Design review of the part built by this model. Coordinates are the model's own, in mm. A direction names the side the tool comes from. Coordinates: 2 decimals unless noted, no trailing zeros. Loops run counter-clockwise (first coordinate to the right, second up) from the corner with the lowest first, then second, coordinate; pieces in that order, holes last. Notation, with made-up numbers: (33.25, 21) -> (45.25, 21) arc R25 cw to (45.25, 46) -> close; hole circle Ø3 at (-21, 30.25). An arc over 180 degrees is marked (long way). Use CSV: the item, a comma, the result in double quotes.
```python
from build123d import *

# Parameters (mm, degrees)
SKETCH1_R           = 12.7
SKETCH1_R_2         = 2
BOSS_EXTRUDE1_DEPTH = 12.7
SKETCH2_W           = 38.1
SKETCH2_H           = 76.2
BOSS_EXTRUDE2_DEPTH = 12.7
FILLET1_R           = 12.7
SKETCH3_W           = 6.35
SKETCH3_H           = 31.75
CUT_EXTRUDE1_DEPTH  = 89.9
BOSS_EXTRUDE3_DEPTH = 38.1
FILLET2_R           = 3.175


with BuildPart() as part:
    # Sketch1 → Boss-Extrude1 (new body)
    # profile 1 of 2: a face of its own
    with BuildSketch(Plane.XY):
        Circle(SKETCH1_R)
        Circle(SKETCH1_R_2, mode=Mode.SUBTRACT)
    # profile 2 of 2: a face of its own
    with BuildSketch(Plane.XY):
        with BuildLine():
            ThreePointArc((12.7, 0), (8.980256121, -8.980256121), (0, -12.7))
            Line((0, -12.7), (25.4, -12.7))
            Line((25.4, -12.7), (25.4, 12.7))
            Line((25.4, 12.7), (0, 12.7))
            ThreePointArc((0, 12.7), (8.980256121, 8.980256121), (12.7, 0))
        make_face()
    extrude(amount=BOSS_EXTRUDE1_DEPTH)

    # Sketch2 → Boss-Extrude2 (add)
    with BuildSketch(Plane(origin=(25.4, 0, 0), x_dir=(0, 0, -1), z_dir=(1, 0, 0))):
        with Locations((-6.35, 0)):
            Rectangle(SKETCH2_W, SKETCH2_H)
    extrude(amount=BOSS_EXTRUDE2_DEPTH)

    # Fillet1
    fillet1_edges = [part.edges().sort_by_distance(p)[0] for p in [
        (25.4, 12.7, 6.35),
        (25.4, -12.7, 6.35),
        (25.4, 0, 12.7),
        (25.4, 0, 0),
    ]]
    fillet(fillet1_edges, radius=FILLET1_R - 0.0001)  # a hair under: the kernel refuses the full size

    # Sketch3 → Cut-Extrude1 (cut, through all)
    with BuildSketch(Plane(origin=(0, 38.1, 0), x_dir=(1, 0, 0), z_dir=(0, 1, 0))):
        with Locations((31.75, -6.35)):
            Rectangle(SKETCH3_W, SKETCH3_H)
    extrude(amount=-CUT_EXTRUDE1_DEPTH, mode=Mode.SUBTRACT)

    # Sketch4 → Boss-Extrude3 (add)
    with BuildSketch(Plane.XY.offset(25.4)):
        with BuildLine():
            Line((38.1, 38.1), (38.1, 25.4))
            ThreePointArc((38.1, 25.4), (44.45, 31.75), (38.1, 38.1))
        make_face()
        with BuildLine():
            Line((38.1, -25.4), (38.1, -38.1))
            ThreePointArc((38.1, -38.1), (44.45, -31.75), (38.1, -25.4))
        make_face()
    extrude(amount=-BOSS_EXTRUDE3_DEPTH)

    # Fillet2
    fillet2_edges = [part.edges().sort_by_distance(p)[0] for p in [
        (34.925, 0, 22.225),
        (28.575, 0, 22.225),
        (34.925, 0, -9.525),
        (28.575, 0, -9.525),
        (38.1, 0, 25.4),
        (38.1, 0, -12.7),
    ]]
    fillet(fillet2_edges, radius=FILLET2_R - 0.0001)  # a hair under: the kernel refuses the full size


solid = part.part
```
Item 1: Add section B-B (y = 0). State how many separate pieces and enclosed holes the cut face has, then the cut area to 3 significant figures.
Checked values:
separate pieces,"2"
enclosed holes,"1"
area,"789 mm^2"
Item 2: To check wall thickness, follow line 1 along X through (y, z) = (18, 3.5) (3 decimals); line 2 along X through (y, z) = (-5, 7) (3 decimals); line 3 along Y through (x, z) = (41.5, 0). State the ranges of each line that lie inside material, in increasing order.
Checked values:
line 1,"23.021 to 28.575, 34.925 to 38.1"
line 2,"-11.674 to 28.575, 34.925 to 38.1"
line 3,"-37.11 to -26.39, 26.39 to 37.11"
Item 3: Add section A-A (z = 3). Give the boundary of the cut face in (x, y) (3 decimals).
Checked values:
outline,"(0, -12.7) -> (12.7, -12.7) arc R12.7 cw to (25.4, -25.4) -> (25.4, -38.1) -> (28.575, -38.1) -> (28.575, 38.1) -> (25.4, 38.1) -> (25.4, 25.4) arc R12.7 cw to (12.7, 12.7) -> (0, 12.7) arc R12.7 ccw to start; (34.925, -38.1) -> (38.1, -38.1) arc R6.35 ccw to (38.1, -25.4) -> (38.1, 25.4) arc R6.35 ccw to (38.1, 38.1) -> (34.925, 38.1) -> close; hole circle Ø4 at (0, 0)"
Item 4: Machinability: for faces 1 (the face through (38.1, 0, 7)), 2 (the face through (33.97, -0.53, 21.32)), 3 (the face through (6, 12.7, 6)), 4 (the face through (6, -12.7, 6)), which of the approach directions +Z, -Z, +X, -X, +Y, -Y give a long, thin tool a straight path to every point of the face, cutting with its end or side? Answer none if there is none.
Checked values:
face 1,"+Z, -Z, +X"
face 2,"+Y, -Y"
face 3,"+Z, -Z, -X, +Y"
face 4,"+Z, -Z, -X, -Y"
Item 5: Draft analysis for pull direction Z (two halves, no side actions). For faces 5 (the face through (23.183, 0.356, -5.53)), 6 (the face through (23.183, -18.23, 6.617)), 7 (the face through (30, -1, -9)), 8 (the face through (37.19, 0.37, 24.45)), state which applies: pulls with the +Z half, pulls with the -Z half, needs draft (parallel to the pull), parting line crosses it, or undercut.
Checked values:
face 5,"pulls with the -Z half"
face 6,"needs draft"
face 7,"undercut"
face 8,"pulls with the +Z half"
Item 6: Add section D-D (z = 20.5). Give the boundary of the cut face in (x, y), then the cut area to 3 significant figures.
Checked values:
outline,"(24.42, -20.5) arc R12.7 cw to (25.4, -25.4) -> (25.4, -38.1) -> (28.93, -38.1) -> (28.93, 38.1) -> (25.4, 38.1) -> (25.4, 25.4) arc R12.7 cw to (24.42, 20.5) -> close; (34.57, -38.1) -> (38.1, -38.1) arc R6.35 ccw to (38.1, -25.4) -> (38.1, 25.4) arc R6.35 ccw to (38.1, 38.1) -> (34.57, 38.1) -> close"
area,"707 mm^2"
Item 7: Add section C-C (x = 33.5). Give the boundary of the cut face in (y, z), then the cut area to 3 significant figures.
Checked values:
outline,"(-38.1, -12.7) -> (38.1, -12.7) -> (38.1, -9) -> (-38.1, -9) -> close; (-38.1, 21.7) -> (38.1, 21.7) -> (38.1, 25.4) -> (-38.1, 25.4) -> close"
area,"564 mm^2"
Item 8: Clearance check with flat-ended pins moving along their axes: pin 1 (1.5 mm diameter, centred on y = 16.5, z = 5, fed in from -X); pin 2 (19 mm diameter, centred on y = 10, z = 14, fed in from -X); pin 3 (7.5 mm diameter, centred on y = 2.5, z = 3, fed in from +X). State where each tip first meets the part, or that it passes through.
Checked values:
pin 1,"x = 20.96"
pin 2,"x = -12.69"
pin 3,"x = 38.1"
